Part model, mm, in its own coordinate system. Face numbers are marked on the shaded views. A direction names the side the tool comes from. Coordinates: 2 decimals unless noted, no trailing zeros. Loops run counter-clockwise (first coordinate to the right, second up) from the corner with the lowest first, then second, coordinate; pieces in that order, holes last. Notation, with made-up numbers: M 69,40 L 109,40 A22 cw 109,72 Z; hole C -20.75,66 d8. An arc over 180 degrees is marked long. Use a Markdown table: item, result. Add a question column.
1) Band-saw the part on D-D (y = 4.5). List the corners of the cut face in (x, z) (3 decimals), plus the area to 4 significant figures.
2) Wall check: probe 1 along Z at (x, y) = (-1.15, 1); probe 2 along Y at (x, z) = (-1.15, 10.5); probe 3 along X at (y, z) = (0.5, 7.5). Give the ranges that are in metal, low to high. Write a range as from..to.
3) Band-saw the part on C-C (z = 12). List the corners of the cut face in (x, y) (3 decimals).
4) Band-saw the part on B-B (y = 0.5). List the corners of the cut face in (x, z) (3 decimals), plus the area to 3 significant figures.
5) Tool access for the marked faces 1 and 2: list every direction of +Z, -Z, +X, -X, +Y, -Y with a clear straight run to the whole face (end or side of a thin tool).
6) Band-saw the part on A-A (x = 0). List the corners of the cut face in (y, z) (3 decimals).
from build123d import *

# Parameters (mm, degrees)
F0_R     = 1.475
F1_DEPTH = 15
F2_W     = 3.95
F2_H     = 7.45
F2_R     = 1.475
F3_DEPTH = 30


with BuildPart() as f1:
    # F0 (on Top) → F1 (new body)
    with BuildSketch(Plane.XY):
        Circle(F0_R)
    extrude(amount=F1_DEPTH)

    # F2 (on face) → F3 (join)
    with BuildSketch(Plane.XY.offset(15)):
        with Locations((0, 1.75)):
            Rectangle(F2_W, F2_H)
        Circle(F2_R, mode=Mode.SUBTRACT)
        Circle(F2_R)
    extrude(amount=F3_DEPTH)


solid = f1.part
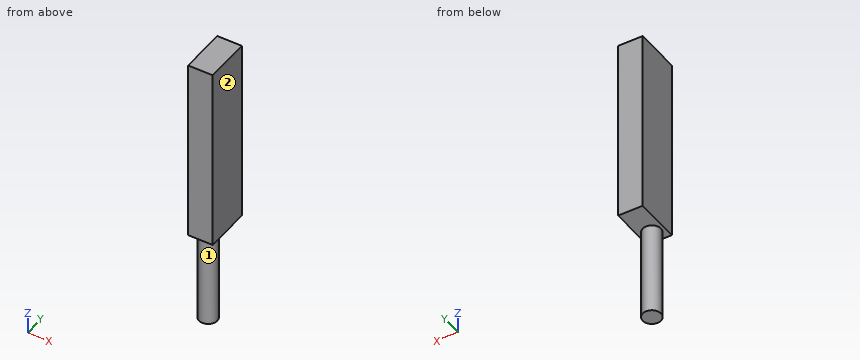
Entries:
| question | item | result |
|---|---|---|
| 1 | outline | M -1.975,15 L 1.975,15 L 1.975,45 L -1.975,45 Z |
| 1 | area | 118.5 mm2 |
| 2 | probe 1 | 15..45 |
| 2 | probe 2 | -0.92..0.92 |
| 2 | probe 3 | -1.39..1.39 |
| 3 | outline | C 0,0 d2.95 |
| 4 | outline | M -1.975,15 L -1.388,15 L -1.388,0 L 1.388,0 L 1.388,15 L 1.975,15 L 1.975,45 L -1.975,45 Z |
| 4 | area | 160 mm2 |
| 5 | face 1 | -Z |
| 5 | face 2 | +Z, -Z, +X, +Y, -Y |
| 6 | outline | M -1.975,15 L -1.475,15 L -1.475,0 L 1.475,0 L 1.475,15 L 5.475,15 L 5.475,45 L -1.975,45 Z |
